from build123d import *

# Parameters (mm, degrees)
F0_W     = 22
F0_H     = 5
F1_DEPTH = 3
F3_DEPTH = 10
F4_R     = 5


with BuildPart() as f1:
    # F0 (on Top) → F1 (new body)
    with BuildSketch(Plane.XY):
        Polygon((49.618883726, 30.5037726198), (-50.381116274, 30.5037726198), (-50.381116274, 3.0037726198), (-50.381116274, -1.9962273802), (-50.381116274, -29.4962273802), (49.618883726, -29.4962273802), align=None)
        with Locations((-61.381116274, 0.5037726198)):
            Rectangle(F0_W, F0_H)
        Polygon((-72.381116274, -1.9962273802), (-72.381116274, 3.0037726198), (-72.381116274, 28.0037726198), (-77.381116274, 28.0037726198), (-77.381116274, -1.9962273802), align=None)
    extrude(amount=F1_DEPTH)

    # F2 (on Right) → F3 (join, symmetric)
    with BuildSketch(Plane.YZ):
        with BuildLine():
            ThreePointArc((-11, -11), (0, 0), (11, -11))
            Line((11, -11), (14, -11))
            ThreePointArc((14, -11), (0, 3), (-14, -11))
            Line((-14, -11), (-11, -11))
        make_face()
    extrude(amount=F3_DEPTH, both=True)

    # F4
    f4_edges = [f1.edges().sort_by_distance(p)[0] for p in [
        (0, -8.660254, 0),
        (0, 8.660254, 0),
    ]]
    fillet(f4_edges, radius=F4_R)


solid = f1.part
Verification items for the finished model (mm, model axes). A direction names the side the tool comes from. Coordinates: 2 decimals unless noted, no trailing zeros. Write each loop counter-clockwise with the first axis right and the second up, starting at its lowest first coordinate (ties: lowest second). Pieces come first, ordered by that corner, then holes. Notation, with made-up numbers: M 24,34.25 L 31,34.25 A19 ccw 31,42.25 Z; hole C -9,52 d11. An arc over 180 degrees is marked long. One line per question, with ' | ' between items.
1) Release check for a two-part mould opening along X. For faces 6 (the face through (-77.381, 13, 1)), 7 (the face through (-62, 3.004, 1)), 8 (the face through (49.619, 0, 1)) record: +X half, -X half, draft (parallel to the pull), parting line (faces both ways), or undercut.
Solutions:
face 6: -X half | face 7: undercut | face 8: +X half
2) Access from +Z, -Z, +X, -X, +Y, -Y to the whole of each face (thin tool, end or side, straight path). Record for faces 1 (the face through (-10, 10, -4)), 2 (the face through (-50.381, 17, 1)), 3 (the face through (-75, 28.004, 1)), 4 (the face through (0.14, -13.815, -8.73)), 5 (the face through (10, -11, -4)).
Solutions:
face 1: -Z, -X, +Y, -Y | face 2: +Z, -Z, +Y | face 3: +Z, -Z, -X, +Y | face 4: +X, -X, -Y | face 5: -Z, +X, +Y, -Y
3) Material ranges on L1, parallel to Z at x = -10.5, y = 3; L2, parallel to X at y = 12.5, z = -1; L3, parallel to Y at x = 8, z = -8.5, recorded low to high.
Solutions:
L1: 0 to 3 | L2: -10 to 10 | L3: -13.77 to -10.71, 10.71 to 13.77
4) Sectioned sample at A-A on y = 24.5. Record the cut outline in (x, z).
Solutions:
outline: M -77.38,0 L -72.38,0 L -72.38,3 L -77.38,3 Z; M -50.38,0 L 49.62,0 L 49.62,3 L -50.38,3 Z
5) Depth check by flat-ended pin: pin 1 Ø1.5 at (x, z) = (-63.5, 2) entering from -Y; pin 2 Ø3.5 at (y, z) = (-6.5, -6) entering from -X; pin 3 Ø1.5 at (x, z) = (-64, 1.5) entering from +Y; pin 4 Ø5.5 at (y, z) = (7.5, -4.5) entering from -X. Enter the tip coordinate at first touch or a pass-through.
Solutions:
pin 1: y = -2 | pin 2: through | pin 3: y = 3 | pin 4: x = -10
6) Sectioned sample at C-C on x = -66.5. Record the cut outline in (y, z).
Solutions:
outline: M -2,0 L 3,0 L 3,3 L -2,3 Z
7) Sectioned sample at B-B on z = -4.5. Record the cut outline in (x, y).
Solutions:
outline: M -10,-13.05 L 10,-13.05 L 10,-8.87 L -10,-8.87 Z; M -10,8.87 L 10,8.87 L 10,13.05 L -10,13.05 Z
8) Sectioned sample at D-D on y = -20. Record the cut outline in (x, z), then the cut area to 3 significant figures.
Solutions:
outline: M -50.38,0 L 49.62,0 L 49.62,3 L -50.38,3 Z | area: 300 mm^2
